Here's how the part is built. I have some questions about the finished solid (model axes, mm). A direction names the side the tool comes from. Give positions to 0.01 mm unless a question says otherwise; leave off trailing zeros. Loops run counter-clockwise (first coordinate to the right, second up) from the corner with the lowest first, then second, coordinate; pieces in that order, holes last. Notation, with made-up numbers: M -23.75,36 L 25.25,36 A29 cw 25.25,67 Z; hole C 18.25,56 d3. An arc over 180 degrees is marked long. Answer as CSV lines item,"result". Start each with the question number.
Item 1: I want a section at B-B on z = 0. List the corners of the cut face in (x, y) for me, plus the area to 3 significant figures.
Item 2: If we mould it in two halves opening along Z, with no side actions, what happens to faces 1 (the cylindrical face through (5.19, 3.98, 9.98)), 2 (the flat face through (14.55, 1.23, 6.53)), 3 (the flat face through (10, 0, 0)), 4 (the cylindrical face through (23.226, 1.232, 0.028))? For each: released by +Z, released by -Z, zero draft, split by the parting line, or undercut.
Item 3: I want a section at A-A on y = 1. List the corners of the cut face in (x, z) for me.
Item 4: If I drill on line 1 along X through (y, z) = (3.25, 0); line 2 along Z through (x, y) = (0, 0.9); line 3 along X through (y, z) = (2.25, 1), over which ranges is the centre line in solid material (lowest first)? Write a range as from..to.
Item 5: I want a section at C-C on x = 0. List the corners of the cut face in (y, z) for me.
Item 6: For faces 5 (the flat face through (0, 2.5, -10)), 6 (the flat face through (4, 6.5, 12)), which set-ups out of +Z, -Z, +X, -X, +Y, -Y let a thin tool reach every point of the face, with its end or its side?
Item 7: Will these pins go through, and if not, where does the flat tip stop? P1, Ø5, axis at x = -17.5, z = -5, coming from the +Y side; P2, Ø3, axis at y = 4, z = 10, coming from the -X side.
Item 8: I want a section at D-D on y = 3.5. List the corners of the cut face in (x, z) for me, plus the area to 3 significant figures.
from build123d import *

# Parameters (mm, degrees)
ESQUISSE1_R        = 2.15
ESQUISSE1_R_2      = 9.75
BOSS_EXTRU_1_DEPTH = 2.5
ESQUISSE2_R        = 13.25
ESQUISSE2_R_2      = 11.25
BOSS_EXTRU_2_DEPTH = 4
CONG_1_R           = 1


with BuildPart() as part:
    # Esquisse1 → Boss.-Extru.1 (new body)
    with BuildSketch(Plane(origin=(0, 0, 0), x_dir=(1, 0, 0), z_dir=(0, 1, 0))):
        with BuildLine():
            Line((-7.0225, 11.23596875), (-22.286415094, 1.695995283))
            ThreePointArc((-22.286415094, 1.695995283), (-23.226415094, 0), (-22.286415094, -1.695995283))
            Line((-22.286415094, -1.695995283), (-7.0225, -11.23596875))
            ThreePointArc((-7.0225, -11.23596875), (0, -13.25), (7.0225, -11.23596875))
            Line((7.0225, -11.23596875), (22.286415094, -1.695995283))
            ThreePointArc((22.286415094, -1.695995283), (23.226415094, 0), (22.286415094, 1.695995283))
            Line((22.286415094, 1.695995283), (7.0225, 11.23596875))
            ThreePointArc((7.0225, 11.23596875), (0, 13.25), (-7.0225, 11.23596875))
        make_face()
        with Locations((-17.305198029, 0)):
            Circle(ESQUISSE1_R, mode=Mode.SUBTRACT)
        Circle(ESQUISSE1_R_2, mode=Mode.SUBTRACT)
        with Locations((18.140226284, 0)):
            Circle(ESQUISSE1_R, mode=Mode.SUBTRACT)
    extrude(amount=BOSS_EXTRU_1_DEPTH)

    # Esquisse2 → Boss.-Extru.2 (add)
    with BuildSketch(Plane(origin=(0, 2.5, 0), x_dir=(1, 0, 0), z_dir=(0, 1, 0))):
        Circle(ESQUISSE2_R)
        Circle(ESQUISSE2_R_2, mode=Mode.SUBTRACT)
    extrude(amount=BOSS_EXTRU_2_DEPTH)

    # Congé1
    cong_1_edges = [part.edges().sort_by_distance(p)[0] for p in [
        (-11.25, 6.5, 0),
    ]]
    fillet(cong_1_edges, radius=CONG_1_R)


solid = part.part
Result:
1,outline,"M -23.23,0 L -19.46,0 L -19.46,2.5 L -23.23,2.5 Z; M -15.16,0 L -9.75,0 L -9.75,2.5 L -11.25,2.5 L -11.25,5.5 A1 ccw -12.25,6.5 L -13.25,6.5 L -13.25,2.5 L -15.16,2.5 Z; M 9.75,0 L 15.99,0 L 15.99,2.5 L 13.25,2.5 L 13.25,6.5 L 12.25,6.5 A1 ccw 11.25,5.5 L 11.25,2.5 L 9.75,2.5 Z; M 20.29,0 L 23.23,0 L 23.23,2.5 L 20.29,2.5 Z"
1,area,"61.5 mm^2"
2,face 1,"undercut"
2,face 2,"released by +Z"
2,face 3,"zero draft"
2,face 4,"split by the parting line"
3,outline,"M -22.29,-1.7 L -7.02,-11.24 A13.25 ccw 7.02,-11.24 L 22.29,-1.7 A2 ccw 22.29,1.7 L 7.02,11.24 A13.25 ccw -7.02,11.24 L -22.29,1.7 A2 ccw Z; hole C -17.31,0 d4.3; hole C 0,0 d19.5; hole C 18.14,0 d4.3"
4,line 1,"-13.25..-11.25, 11.25..13.25"
4,line 2,"-13.25..-9.75, 9.75..13.25"
4,line 3,"-22.96..-19.21, -15.4..-9.7, 9.7..16.24, 20.04..22.96"
5,outline,"M 0,-13.25 L 6.5,-13.25 L 6.5,-12.25 A1 ccw 5.5,-11.25 L 2.5,-11.25 L 2.5,-9.75 L 0,-9.75 Z; M 0,9.75 L 2.5,9.75 L 2.5,11.25 L 5.5,11.25 A1 ccw 6.5,12.25 L 6.5,13.25 L 0,13.25 Z"
6,face 5,"+Y"
6,face 6,"+Z, -Z, +X, -X, +Y"
7,P1,"y = 2.5"
7,P2,"x = -10.16"
8,outline,"C 0,0 d26.5; hole C 0,0 d22.5"
8,area,"154 mm^2"
